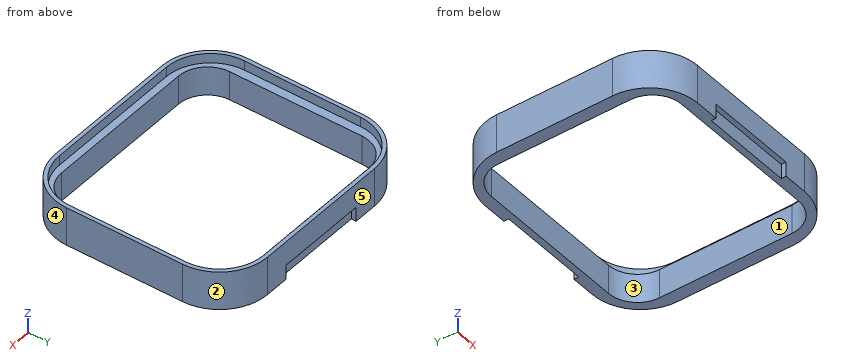
from build123d import *

# Parameters (mm, degrees)
F1_DEPTH = 8
F3_DEPTH = 8.001
F5_DEPTH = 2
F6_W     = 19
F6_H     = 1
F7_DEPTH = 3
F8_W     = 19
F8_H     = 1
F9_DEPTH = 3


with BuildPart() as f1:
    # F0 (on Top) → F1 (new body)
    with BuildSketch(Plane.XY):
        with BuildLine():
            Line((-14.5, -22.05), (14.5, -22.05))
            ThreePointArc((14.5, -22.05), (21.5710678119, -19.1210678119), (24.5, -12.05))
            Line((24.5, -12.05), (24.5, 12.05))
            ThreePointArc((24.5, 12.05), (21.5710678119, 19.1210678119), (14.5, 22.05))
            Line((14.5, 22.05), (-14.5, 22.05))
            ThreePointArc((-14.5, 22.05), (-21.5710678119, 19.1210678119), (-24.5, 12.05))
            Line((-24.5, 12.05), (-24.5, -12.05))
            ThreePointArc((-24.5, -12.05), (-21.5710678119, -19.1210678119), (-14.5, -22.05))
        make_face()
    extrude(amount=F1_DEPTH)

    # F2 (on face) → F3 (cut, through all)
    with BuildSketch(Plane.XY.offset(8)):
        with BuildLine():
            Line((-15.9, -19.75), (15.9, -19.75))
            ThreePointArc((15.9, -19.75), (20.1426406871, -17.9926406871), (21.9, -13.75))
            Line((21.9, -13.75), (21.9, 13.75))
            ThreePointArc((21.9, 13.75), (20.1426406871, 17.9926406871), (15.9, 19.75))
            Line((15.9, 19.75), (-15.9, 19.75))
            ThreePointArc((-15.9, 19.75), (-20.1426406871, 17.9926406871), (-21.9, 13.75))
            Line((-21.9, 13.75), (-21.9, -13.75))
            ThreePointArc((-21.9, -13.75), (-20.1426406871, -17.9926406871), (-15.9, -19.75))
        make_face()
    extrude(amount=-F3_DEPTH, mode=Mode.SUBTRACT)

    # F4 (on face) → F5 (cut)
    with BuildSketch(Plane.XY.offset(8)):
        with BuildLine():
            ThreePointArc((14.5, -21.25), (21.0053823869, -18.5553823869), (23.7, -12.05))
            Line((23.7, -12.05), (23.7, 12.05))
            ThreePointArc((23.7, 12.05), (21.0053823869, 18.5553823869), (14.5, 21.25))
            Line((14.5, 21.25), (-14.5, 21.25))
            ThreePointArc((-14.5, 21.25), (-21.0053823869, 18.5553823869), (-23.7, 12.05))
            Line((-23.7, 12.05), (-23.7, -12.05))
            ThreePointArc((-23.7, -12.05), (-21.0053823869, -18.5553823869), (-14.5, -21.25))
            Line((-14.5, -21.25), (14.5, -21.25))
        make_face()
    extrude(amount=-F5_DEPTH, mode=Mode.SUBTRACT)

    # F6 (on Top) → F7 (cut)
    with BuildSketch(Plane.XY):
        with Locations((0, -21.55)):
            Rectangle(F6_W, F6_H)
    extrude(amount=F7_DEPTH, mode=Mode.SUBTRACT)

    # F8 (on face) → F9 (cut)
    with BuildSketch(Plane(origin=(0, 0, 0), x_dir=(1, 0, 0), z_dir=(0, 0, -1))):
        with Locations((0, -21.55)):
            Rectangle(F8_W, F8_H)
    extrude(amount=-F9_DEPTH, mode=Mode.SUBTRACT)


solid = f1.part
Could you check a few things on this model? Use its own coordinates, in mm. Face numbers are marked on the shaded views. A direction names the side the tool comes from. Coordinates: 2 decimals unless noted, no trailing zeros. Order: outer loops, then holes, each group sorted by start corner. A loop starts at its lowest first (then second) coordinate and runs counter-clockwise, first axis right, second up.
Q1. Suppose I cut it at C-C on y = -10. Please give me the cut outline in (x, z).
Q2. Suppose I cut it at D-D on z = 2. Please give me the cut outline in (x, y).
Q3. Will these pins go through, and if not, where does the flat tip stop? pin 1 (0.8 mm diameter, centred on y = -21.5, z = 2, fed in from +X); pin 2 (5 mm diameter, centred on x = 18.5, y = 6, fed in from -Z); pin 3 (0.5 mm diameter, centred on x = -1, y = -21.5, fed in from -Z); pin 4 (1.1 mm diameter, centred on y = -21.5, z = 1.5, fed in from -X).
Q4. Suppose I cut it at A-A on x = 2. Please give me the cut outline in (y, z), and give its area (3 significant figures).
Q5. Thinking about a two-plate mould opening in X: for the marked faces 3, 4 and 5, which applies, released by +X, released by -X, zero draft, split by the parting line, or undercut?
Q6. Which directions (+Z, -Z, +X, -X, +Y, -Y) give clear straight access to the entire face, cutting with the end or side of a thin tool? Please do the marked faces 1 and 2.
Q7. Suppose I cut it at B-B on z = 4.5. Please give me the cut outline in (x, y), and give its area (3 significant figures).
Q8. Please list where these lines run through material, in increasing order: L1, parallel to Y at x = 6.5, z = 7.5; L2, parallel to X at y = -10, z = 4; L3, parallel to Y at x = 13.5, z = 5.25.
Answer:
1. outline: (-24.5, 0) - (-21.9, 0) - (-21.9, 6) - (-23.7, 6) - (-23.7, 8) - (-24.5, 8) - close; (21.9, 0) - (24.5, 0) - (24.5, 8) - (23.7, 8) - (23.7, 6) - (21.9, 6) - close
2. outline: (-24.5, -12.05) arc R10 ccw to (-14.5, -22.05) - (-9.5, -22.05) - (-9.5, -21.05) - (9.5, -21.05) - (9.5, -22.05) - (14.5, -22.05) arc R10 ccw to (24.5, -12.05) - (24.5, 12.05) arc R10 ccw to (14.5, 22.05) - (9.5, 22.05) - (9.5, 21.05) - (-9.5, 21.05) - (-9.5, 22.05) - (-14.5, 22.05) arc R10 ccw to (-24.5, 12.05) - close; hole (-21.9, -13.75) arc R6 ccw to (-15.9, -19.75) - (15.9, -19.75) arc R6 ccw to (21.9, -13.75) - (21.9, 13.75) arc R6 ccw to (15.9, 19.75) - (-15.9, 19.75) arc R6 ccw to (-21.9, 13.75) - close
3. pin 1: stops at x = 18.75
3. pin 2: passes through
3. pin 3: stops at z = 3
3. pin 4: stops at x = -19.06
4. outline: (-22.05, 3) - (-21.05, 3) - (-21.05, 0) - (-19.75, 0) - (-19.75, 6) - (-21.25, 6) - (-21.25, 8) - (-22.05, 8) - close; (19.75, 0) - (21.05, 0) - (21.05, 3) - (22.05, 3) - (22.05, 8) - (21.25, 8) - (21.25, 6) - (19.75, 6) - close
4. area: 24.8 mm2
5. face 3: undercut
5. face 4: released by +X
5. face 5: zero draft
6. face 1: +Z, -Z
6. face 2: +Z, -Z, +X, +Y
7. outline: (-24.5, -12.05) arc R10 ccw to (-14.5, -22.05) - (14.5, -22.05) arc R10 ccw to (24.5, -12.05) - (24.5, 12.05) arc R10 ccw to (14.5, 22.05) - (-14.5, 22.05) arc R10 ccw to (-24.5, 12.05) - close; hole (-21.9, -13.75) arc R6 ccw to (-15.9, -19.75) - (15.9, -19.75) arc R6 ccw to (21.9, -13.75) - (21.9, 13.75) arc R6 ccw to (15.9, 19.75) - (-15.9, 19.75) arc R6 ccw to (-21.9, 13.75) - close
7. area: 376 mm2
8. L1: y = -22.05 to -21.25, 21.25 to 22.05
8. L2: x = -24.5 to -21.9, 21.9 to 24.5
8. L3: y = -22.05 to -19.75, 19.75 to 22.05
